For this review, take the finished solid that the model builds, in its own axes (mm). A direction names the side the tool comes from. Round coordinates to 2 decimals unless told otherwise and drop trailing zeros. Write each loop counter-clockwise with the first axis right and the second up, starting at its lowest first coordinate (ties: lowest second). Pieces come first, ordered by that corner, then holes. Notation, with made-up numbers: (45.5, -23) -> (81.5, -23) arc R18 ccw to (81.5, -7) -> close; hole circle Ø11 at (60, 87). An arc over 180 degrees is marked (long way). Write each question's results on one line, items separated by ' | '. Start each with the question number.
Item 1: To check wall thickness, follow line 1 along Z through (x, y) = (260.5, -167); line 2 along Y through (x, z) = (-194, -58); line 3 along Y through (x, z) = (85.5, -75). State the ranges of each line that lie inside material, in increasing order.
Item 2: Add section A-A (x = -218). State the section outline as (y, z) points, plus the area to 3 significant figures.
Item 3: Add section C-C (z = -108.5). State the section outline as (x, y) points.
Item 4: Add section B-B (y = 33). State the section outline as (x, z) points, plus the area to 3 significant figures.
Item 5: Clearance check with flat-ended pins moving along their axes: pin 1 (8 mm diameter, centred on x = 79, z = -15, fed in from -Y); pin 2 (12 mm diameter, centred on x = -165.5, y = -629, fed in from -Z); pin 3 (12 mm diameter, centred on x = -148, z = -128.5, fed in from +Y). State where each tip first meets the part, or that it passes through.
Item 6: Tool access review of faces 1 (the flat face through (-4, 15, 0)), 2 (the flat face through (-4, -1027, -74)): name each direction out of +Z, -Z, +X, -X, +Y, -Y from which nothing blocks a thin tool from reaching the whole face with its end or side.
Autodesk Inventor part; units mm, degrees
ref_plane "YZ Plane" through (0, 0, 0) normal (1, 0, 0) x (0, 1, 0)
ref_plane "XZ Plane" through (0, 0, 0) normal (0, 1, 0) x (-1, 0, 0)
ref_plane "XY Plane" through (0, 0, 0) normal (0, 0, 1) x (1, 0, 0)
sketch "Sketch1" plane through (0, 0, 0) normal (0, 0, 1) x (1, 0, 0)
  line L0 (-300, -950) -> (300, -950)
  line L1 (300, -950) -> (300, 950)
  line L2 (300, 950) -> (-300, 950)
  line L3 (-300, 950) -> (-300, -950)
  line L4 (-300, -950) -> (300, 950) construction
  line L5 (300, -950) -> (-300, 950) construction
  point P0 (0, 0)
  dimension "d0" = 600
  dimension "d1" = 1900
extrude "Plate1" add sketch "Sketch1" along normal blind 3
sketch "Sketch3" plane through (-300, -947.8787, 0.8787) normal (0, -0.7071068, 0.7071068) x (1, 0, 0)
  line L0 (600, 0) -> (0, 0)
  line L1 (0, 0) -> (0, -212)
  line L2 (0, -212) -> (600, -212)
  line L3 (600, -212) -> (600, 0)
edge flange "Flange2" height 212 angle 45 thickness 3 bend radius 5 thickness toward (0, -0.7071068, 0.7071068) relief round relief width 3 relief depth 1.5 edges at (0, -950, 0) wall of the first edge with corners at (300, -947.8787, 0.8787) (-300, -947.8787, 0.8787) (-300, -1097.7853, -149.028) (300, -1097.7853, -149.028)
bend "Bend2"
corner "Corner2"
sketch "Sketch5" plane through (300, -1097.7853, -149.028) normal (0, 0.7071068, -0.7071068) x (-1, 0, 0)
  line L0 (575, 36.661) -> (575, 25) construction
  line L1 (575, 25) -> (375, 25) construction
  line L2 (375, 25) -> (375, 36.661) construction
  line L3 (375, 36.661) -> (575, 36.661) construction
  line L4 (0, 0) -> (600, 0)
  line L5 (600, 208.6863) -> (600, 0)
  point P0 (300, 881.6301)
  point P1 (575, 30.8305)
  dimension "d23" = 200
  dimension "d24" = 11.661
  dimension "d25" = 25
  dimension "d26" = 25
mark "Mark1"
equation "\"d2\" = Thickness"
equation "\"d13\" = BendReliefWidth"
equation "\"d14\" = BendReliefDepth"
equation "\"d15\" = MinimumRemnant"
equation "\"d16\" = TransitionRadius"
equation "\"d19\" = BendRadius"
equation "\"d20\" = CornerReliefSize"
equation "\"d21\" = GapSize"
equation "\"d22\" = JacobiRadiusSize"
equation "\"BendReliefWidth\" = Thickness"
equation "\"BendReliefDepth\" = 0.5 * Thickness"
equation "\"CornerReliefSize\" = 4 * Thickness"
equation "\"MinimumRemnant\" = 2 * Thickness"
equation "\"TransitionRadius\" = BendRadius"
equation "\"JacobiRadiusSize\" = BendRadius"
equation "\"GapSize\" = Thickness"
properties part number "BSH 013 floor" material "09g2s"
Responses:
1) line 1: z = 0 to 3 | line 2: y = -1011 to -1006.76 | line 3: y = -1028 to -1023.76
2) outline: (-1099.91, -146.91) -> (-1097.79, -149.03) -> (-950.22, -1.46) arc R5 cw to (-946.69, 0) -> (950, 0) -> (950, 3) -> (-946.69, 3) arc R8 ccw to (-952.34, 0.66) -> close | area: 6,330 mm^2
3) outline: (-300, -1061.5) -> (300, -1061.5) -> (300, -1057.26) -> (-300, -1057.26) -> close
4) outline: (-300, 0) -> (300, 0) -> (300, 3) -> (-300, 3) -> close | area: 1,800 mm^2
5) pin 1: stops at y = -972 | pin 2: stops at z = 0 | pin 3: stops at y = -1071.26
6) face 1: -Z, +X, -X, +Y | face 2: +Z, +X, -X, -Y
